Can you work these out from the model? Positions are in its coordinate system, mm. A direction names the side the tool comes from. Round coordinates to 2 decimals unless told otherwise and drop trailing zeros. Loops run counter-clockwise (first coordinate to the right, second up) from the corner with the lowest first, then second, coordinate; pieces in that order, holes last. Notation, with made-up numbers: (0.5, -29.5) -> (28.5, -29.5) arc R19 ccw to (28.5, -1.5) -> close; hole circle Ø1 at (74, 42). An arc over 180 degrees is marked (long way). Use a Markdown table: item, result.
Autodesk Inventor part; units mm, degrees
ref_plane "XY Plane" through (0, 0, 0) normal (0, 0, 1) x (1, 0, 0)
sketch "Sketch1" plane through (0, 0, 0) normal (1, 0, 0) x (0, 1, 0)
  line L0 (0, -8.89) -> (0, -1.27)
  line L1 (0, -1.27) -> (0, -8.89)
  line L2 (0, -1.27) -> (-10.16, -1.27)
  line L3 (-10.16, -8.89) -> (0, -8.89)
  line L4 (0, -8.89) -> (0, -1.27)
  line L5 (-31.4325, -3.175) -> (-10.16, -3.175)
  line L6 (-10.16, -6.985) -> (-31.4325, -6.985)
  line L7 (-10.16, -1.27) -> (-10.16, -3.175)
  line L8 (-10.16, -6.985) -> (-10.16, -8.89)
  line L9 (-31.4325, -3.175) -> (-31.4325, 0)
  line L10 (-31.4325, 0) -> (-36.5125, 0)
  line L11 (-36.5125, 0) -> (-36.5125, -10.16)
  line L12 (-31.4325, -6.985) -> (-31.4325, -10.16)
  line L13 (-31.4325, -10.16) -> (-36.5125, -10.16)
  dimension "d11" = 10.16
  dimension "d16" = 21.2725
  dimension "d17" = 21.2725
  dimension "d18" = 5.08
  dimension "d19" = 10.16
revolve "Revolution1" add sketch "Sketch1" angle 360 about axis through (0, 0, -8.89) along (0, 0, 1)
sketch "Sketch2" plane through (0, 0, -1.27) normal (0, 0, 1) x (1, 0, 0)
  line L0 (0, 0) -> (0, 6.35)
  line L1 (3.6662, 6.35) -> (7.3323, 0)
  line L2 (7.3323, 0) -> (3.6662, -6.35)
  line L3 (3.6662, -6.35) -> (-3.6662, -6.35)
  line L4 (-3.6662, -6.35) -> (-7.3323, 0)
  line L5 (-7.3323, 0) -> (-3.6662, 6.35)
  line L6 (-3.6662, 6.35) -> (3.6662, 6.35)
  circle A0 centre (0, 0) radius 36.5125
  circle A1 centre (0, 0) radius 31.4325
  dimension "d12" = 6.35
  dimension "d20" = 6.35
extrude "Extrusion1" cut sketch "Sketch2" against normal blind 25.4 contours L1 L2 L3 L4 L5 L6
ref_plane "Work Plane1" through (0, 0, 0) normal (1, 0, 0) x (0, 1, 0)
ref_plane "Work Plane2" through (0, 0, 0) normal (0, 1, 0) x (-1, 0, 0)
properties part number "BaneBots_Wheel"
1. I want a section at D-D (x = 25.5). Please give me the cut outline in (y, z) (3 decimals).
Answer sheet:
| item | result |
|---|---|
| outline | (-26.133, -10.16) -> (-18.378, -10.16) -> (-18.378, -6.985) -> (18.378, -6.985) -> (18.378, -10.16) -> (26.133, -10.16) -> (26.133, 0) -> (18.378, 0) -> (18.378, -3.175) -> (-18.378, -3.175) -> (-18.378, 0) -> (-26.133, 0) -> close |
2. I want a section at C-C (y = -12.5). Please give me the cut outline in (x, z) (3 decimals).
Answer sheet:
| item | result |
|---|---|
| outline | (-34.306, -10.16) -> (-28.84, -10.16) -> (-28.84, -6.985) -> (28.84, -6.985) -> (28.84, -10.16) -> (34.306, -10.16) -> (34.306, 0) -> (28.84, 0) -> (28.84, -3.175) -> (-28.84, -3.175) -> (-28.84, 0) -> (-34.306, 0) -> close |
3. If we mould it in two halves opening along Y, with no side actions, what happens to faces 5 (the cylindrical face through (-10.967, -34.826, -5.151)), 6 (the flat face through (27.2, -16.1, 0)), 7 (the cylindrical face through (-10.074, 1.323, -7.951))? For each: +Y half, -Y half, draft (parallel to the pull), parting line (faces both ways), or undercut.
Answer sheet:
| item | result |
|---|---|
| face 5 | parting line |
| face 6 | draft |
| face 7 | undercut |
4. Which directions (+Z, -Z, +X, -X, +Y, -Y) give clear straight access to the entire face, cutting with the end or side of a thin tool? Please do faces 1 (the flat face through (0, -6.35, -5)), 2 (the flat face through (7.4, 7.4, -3.175)), 3 (the cylindrical face through (19.13, 24.94, -8.59)), 4 (the flat face through (27.2, -16.1, -10.16)).
Answer sheet:
| item | result |
|---|---|
| face 1 | +Z, -Z |
| face 2 | +Z |
| face 3 | -Z |
| face 4 | -Z, +X, -X, +Y, -Y |
5. I need wall thicknesses on line 1 (X direction, y = 0, z = -2.2); line 2 (Y direction, x = -1.5, z = -8.75); line 3 (Y direction, x = -9, z = -1.75). Which ranges of each line are inside material? Lowest first, please.
Answer sheet:
| item | result |
|---|---|
| line 1 | x = -36.51 to -31.43, -10.16 to -7.33, 7.33 to 10.16, 31.43 to 36.51 |
| line 2 | y = -36.48 to -31.4, -10.05 to -6.35, 6.35 to 10.05, 31.4 to 36.48 |
| line 3 | y = -35.39 to -30.12, -4.71 to 4.71, 30.12 to 35.39 |
6. Will these pins go through, and if not, where does the flat tip stop? pin 1 Ø2 at (x, y) = (-16.5, -19.5) entering from +Z (3 decimals); pin 2 Ø5 at (y, z) = (20, -8.5) entering from -X; pin 3 Ø10 at (x, y) = (-5, 4.5) entering from +Z.
Answer sheet:
| item | result |
|---|---|
| pin 1 | stops at z = -3.175 |
| pin 2 | stops at x = -32.05 |
| pin 3 | stops at z = -1.27 |
